Source: three-view drawing plus pictorial views. Frame: mm from the lowest corner of the part. A direction names the side the tool comes from. Round coordinates to 2 decimals unless told otherwise and drop trailing zeros. Loops run counter-clockwise (first coordinate to the right, second up) from the corner with the lowest first, then second, coordinate; pieces in that order, holes last. Notation, with made-up numbers: M -1.75,-15.5 L 12.25,-15.5 A18 cw 12.25,5.5 Z; hole C -7,32.5 d2. An arc over 180 degrees is marked long. Return JSON: item names as keys, results as strings. Group by question number.
1) Contact query for flat-ended pins moving along their axis: P1, Ø2, axis at x = 27, z = 10, coming from the +Y side; P2, Ø12, axis at x = 30, z = 17, coming from the -Y side; P3, Ø4, axis at x = 35, z = 20.5, coming from the +Y side; P4, Ø5, axis at x = 18, y = 37, coming from the -Z side. Output: stop coordinate, or through.
2) Mould query, pull axis X, two halves, no side actions, for the marked faces 1, 2, 3 and 4. Classes: +X half, -X half, draft (parallel to the pull), parting line (faces both ways), or undercut.
3) Section A-A (x = 30). Output: boundary loops of the cut face in (y, z).
4) Material intervals for line 1 (X direction, y = 46.5, z = 21.75); line 2 (Y direction, x = 31.5, z = 7); line 3 (Y direction, x = 13, z = 14.75) (1 decimal), sorted ascending. Write a range as from..to.
5) Access query for the marked faces 5 and 6. Directions: +Z, -Z, +X, -X, +Y, -Y. A direction counts if a zero-diameter tool reaches every point of the face in a straight line with its end or side. Return the directions, or none.
6) Section C-C (z = 2). Output: boundary loops of the cut face in (x, y) (1 decimal), plus the area to 3 significant figures.
7) Section B-B (y = 64.5). Output: boundary loops of the cut face in (x, z).
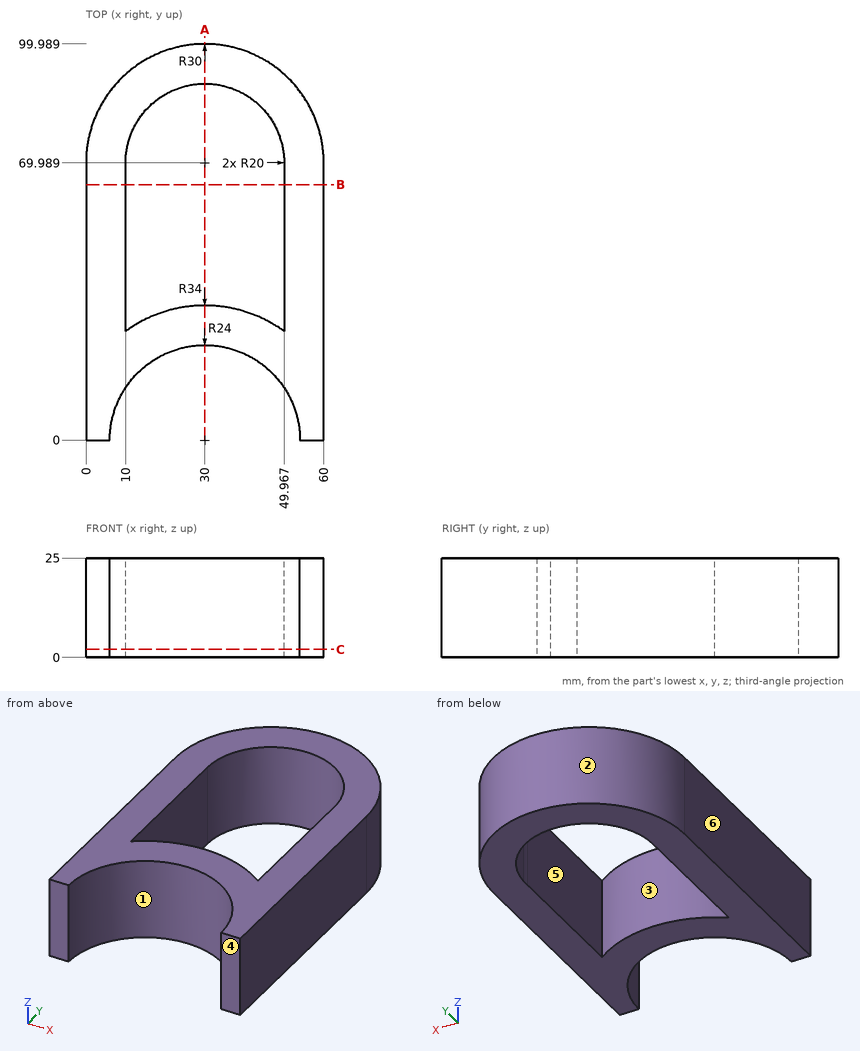
Returned:
{
 "1": {"P1": "stops at y = 99.92", "P2": "stops at y = 23.24", "P3": "stops at y = 99.84", "P4": "passes through"},
 "2": {"face 1": "undercut", "face 2": "parting line", "face 3": "undercut", "face 4": "draft"},
 "3": {"outline": "M 24,0 L 34,0 L 34,25 L 24,25 Z; M 89.99,0 L 99.99,0 L 99.99,25 L 89.99,25 Z"},
 "4": {"line 1": "x = 0..10, 49.97..60", "line 2": "y = 23.95..33.97, 89.93..99.95", "line 3": "y = 16.9..29.4, 80.5..94.7"},
 "5": {"face 5": "+Z, -Z", "face 6": "+Z, -Z, -X, +Y, -Y"},
 "6": {"outline": "M 0,0 L 6,0 A24 cw 54,0 L 60,0 L 60,70 A30 ccw 0,70 Z; hole M 10,27.5 A34 cw 50,27.5 L 50,68.8 A20 ccw 50,71.1 A20 ccw 10,70 Z", "area": "2,560 mm^2"},
 "7": {"outline": "M 0,0 L 10,0 L 10,25 L 0,25 Z; M 49.97,0 L 60,0 L 60,25 L 49.97,25 Z"}
}
